Autodesk Inventor part; units mm, degrees
ref_plane "YZ Plane" through (0, 0, 0) normal (1, 0, 0) x (0, 1, 0)
ref_plane "XZ Plane" through (0, 0, 0) normal (0, 1, 0) x (-1, 0, 0)
ref_plane "XY Plane" through (0, 0, 0) normal (0, 0, 1) x (1, 0, 0)
sketch "Sketch2" plane through (0, 0, 0) normal (0, 0, 1) x (1, 0, 0)
  line L0 (-17, 0) -> (17, 0)
  line L1 (-17, 0) -> (-17, -4)
  line L2 (-17, -4) -> (-14.5, -4)
  line L3 (-14.5, -4) -> (-13, -2.5)
  line L4 (-13, -2.5) -> (-11.5, -4)
  line L5 (-11.5, -4) -> (0, -4)
  line L6 (0, 0) -> (0, -4) construction
  line L7 (-13, -2.5) -> (-13, 0) construction
  line L8 (17, 0) -> (17, -4)
  line L9 (17, -4) -> (14.5, -4)
  line L10 (14.5, -4) -> (13, -2.5)
  line L11 (13, -2.5) -> (11.5, -4)
  line L12 (11.5, -4) -> (0, -4)
  dimension "d1" = 34
  dimension "d2" = 135
  dimension "d3" = 4
  dimension "d4" = 8
  dimension "d5" = 3
revolve "Revolution1" add sketch "Sketch2" angle 360 about axis through (-17, 0, 0) along (1, 0, 0)
chamfer "Chamfer1" distance 0.2 angle 45 2 edges at (-17, 4, 0) (17, 4, 0)
properties part number "TL20240701-10100AT-002" material "S45C"
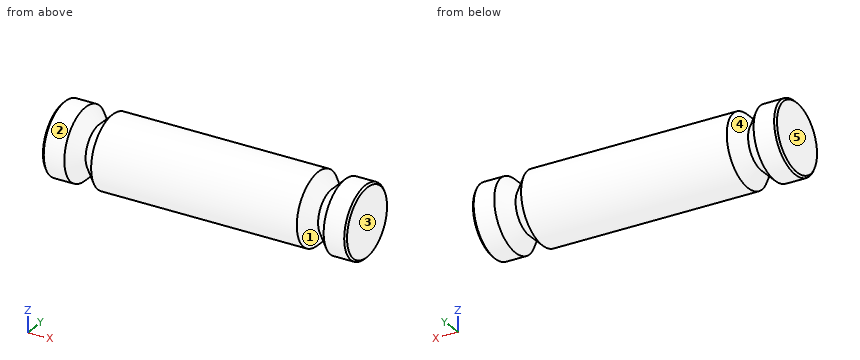
The listing builds one solid part. Answer for the finished solid, in the listing's coordinates (mm). Face numbers are marked on the shaded views. A direction names the side the tool comes from. Coordinates: 2 decimals unless noted, no trailing zeros. Order: outer loops, then holes, each group sorted by start corner. A loop starts at its lowest first (then second) coordinate and runs counter-clockwise, first axis right, second up. Notation, with made-up numbers: M -37,30.5 L 17,30.5 A25 ccw 17,52.5 Z; hole C 53.25,9.25 d4. An arc over 180 degrees is marked long. Answer as a JSON object with one key per item and string values. Group by question number.
1. Section C-C on x = 1.5 is taken. Write down the section's boundary in (y, z).
2. Section A-A on y = 0 is taken. Write down the section's boundary in (x, z), then the cut area to 3 significant figures.
3. Determine the mould class of the marked faces 1, 2 and 3 for opening direction X: released by +X, released by -X, zero draft, split by the parting line, or undercut.
4. Flat-ended cylindrical pins translate along their axes: P1, Ø2, axis at x = 2, z = -2, coming from the -Y side; P2, Ø2, axis at x = -9, y = 1.5, coming from the +Z side. Find the tip coordinate at first contact, or state that the pin passes through.
5. A tool of negligible diameter and unlimited length cuts with its end or side. For the marked faces 4 and 5, from which of +Z, -Z, +X, -X, +Y, -Y can it reach the whole face along a straight path? Write none if from no direction.
6. Straight lines are drawn through the part: line 1 (X direction, y = 1.5, z = -2.5); line 2 (X direction, y = -2, z = -2); line 3 (Y direction, x = 10.5, z = 0.25). For each, find the intervals that lie inside material, in ascending order.
7. Section D-D on z = -3.25 is taken. State how many separate pieces and enclosed holes the cut face has, then the cut area to 3 significant figures.
Values follow:
{
 "1": {"outline": "C 0,0 d8"},
 "2": {"outline": "M -17,-3.8 L -16.8,-4 L -14.5,-4 L -13,-2.5 L -11.5,-4 L 11.5,-4 L 13,-2.5 L 14.5,-4 L 16.8,-4 L 17,-3.8 L 17,3.8 L 16.8,4 L 14.5,4 L 13,2.5 L 11.5,4 L -11.5,4 L -13,2.5 L -14.5,4 L -16.8,4 L -17,3.8 Z", "area": "263 mm2"},
 "3": {"face 1": "undercut", "face 2": "zero draft", "face 3": "released by +X"},
 "4": {"P1": "y = -3.87", "P2": "z = 3.97"},
 "5": {"face 4": "none", "face 5": "+Z, -Z, -X, +Y, -Y"},
 "6": {"line 1": "-17 to -13.42, -12.58 to 12.58, 13.42 to 17", "line 2": "-17 to -13.33, -12.67 to 12.67, 13.33 to 17", "line 3": "-3.99 to 3.99"},
 "7": {"separate pieces": "3", "enclosed holes": "0", "area": "140 mm2"}
}
